Geometry: final body of the model. Coordinates: model frame, mm. A direction names the side the tool comes from. Round coordinates to 2 decimals unless told otherwise and drop trailing zeros. Order: outer loops, then holes, each group sorted by start corner. A loop starts at its lowest first (then second) coordinate and runs counter-clockwise, first axis right, second up. Notation, with made-up numbers: (15, -38.75) - (39, -38.75) arc R25 cw to (39, -12.75) - close; hole circle Ø8 at (-1, 14.25). An arc over 180 degrees is marked (long way). Put each result on its own line as item: value. Start each with the question number.
(1) Section C-C (z = 64). Output: boundary loops of the cut face in (x, y).
(2) Section D-D (x = 7). Output: boundary loops of the cut face in (y, z), and give its area (3 significant figures).
(3) Pull-direction query (X, two-part tool) for faces 1 (the face through (22.377, -63, 69)), 2 (the face through (67, -63, 22.86)), 3 (the face through (77.435, -63, 11)); classes: released by +X, released by -X, zero draft, split by the parting line, or undercut.
(4) Section B-B (x = 61). Output: boundary loops of the cut face in (y, z), and give its area (3 significant figures).
(5) Pin query (flat end, axial travel): P1, Ø7.5, axis at y = -72.5, z = 65.5, coming from the +X side; P2, Ø23, axis at x = 25, z = 38.5, coming from the -Y side; P3, Ø12.5, axis at y = -14.5, z = 49.5, coming from the +X side; P4, Ø1, axis at y = -26.5, z = 29.5, coming from the -X side. Return the tip coordinate at first contact, or that it passes through.
(6) Material intervals for L1, parallel to Z at x = 73.5, y = -66; L2, parallel to X at y = -58, z = 8.5; L3, parallel to Z at x = 9, y = -45, sorted ascending. Write a range as [from, to].
(7) Section A-A (y = -40.5). Output: boundary loops of the cut face in (x, z), and give its area (3 significant figures).
(8) Access query for faces 4 (the face through (24.278, -63, 10)), 5 (the face through (58.223, -63, 68)), 6 (the face through (13, -63, 20.32)), 7 (the face through (68, -63, 76.113)), 8 (the face through (68, -63, 60.945)). Directions: +Z, -Z, +X, -X, +Y, -Y. A direction counts if a zero-diameter tool reaches every point of the face in a straight line with its end or side. Return the directions, or none.
from build123d import *

# Parameters (mm, degrees)
F0_W     = 75.953597
F0_H     = 76.343752
F1_DEPTH = 25.4
F2_W     = 22.86
F2_H     = 20.32
F2_W_2   = 20.958833
F2_H_2   = 15.39883
F3_DEPTH = 76.2
F5_W     = 20.32
F5_H     = 22.86
F5_W_2   = 19.010187
F5_H_2   = 15.167706
F6_DEPTH = 76.2


with BuildPart() as f1:
    # F0 (on Front) → F1 (new body)
    with BuildSketch(Plane.XZ):
        with Locations((39.394597, 38.171876)):
            Rectangle(F0_W, F0_H)
    extrude(amount=F1_DEPTH)

    # F2 (on face) → F3 (join)
    with BuildSketch(Plane.XZ.offset(25.4)):
        with Locations((12.847799, 10.16)):
            Rectangle(F2_W, F2_H)
        with Locations((11.897215, 68.644337)):
            Rectangle(F2_W_2, F2_H_2)
    extrude(amount=F3_DEPTH)

    # F5 (on face) → F6 (join)
    with BuildSketch(Plane.XZ.offset(25.4)):
        with Locations((67.275393, 11.43)):
            Rectangle(F5_W, F5_H)
        with Locations((67.728057, 68.528775)):
            Rectangle(F5_W_2, F5_H_2)
    extrude(amount=F6_DEPTH)


solid = f1.part
Checks:
1. outline: (1.42, -101.6) - (22.38, -101.6) - (22.38, -25.4) - (58.22, -25.4) - (58.22, -101.6) - (77.23, -101.6) - (77.23, -25.4) - (77.37, -25.4) - (77.37, 0) - (1.42, 0) - close
2. outline: (-101.6, 0) - (0, 0) - (0, 76.34) - (-101.6, 76.34) - (-101.6, 60.94) - (-25.4, 60.94) - (-25.4, 20.32) - (-101.6, 20.32) - close
2. area: 4,660 mm²
3. face 1: undercut
3. face 2: zero draft
3. face 3: released by +X
4. outline: (-101.6, 0) - (0, 0) - (0, 76.34) - (-25.4, 76.34) - (-25.4, 76.11) - (-101.6, 76.11) - (-101.6, 60.94) - (-25.4, 60.94) - (-25.4, 22.86) - (-101.6, 22.86) - close
4. area: 4,840 mm²
5. P1: stops at x = 77.23
5. P2: stops at y = -25.4
5. P3: stops at x = 77.37
5. P4: passes through
6. L1: z = [0, 22.86], [60.94, 76.11]
6. L2: x = [1.42, 24.28], [57.12, 77.44]
6. L3: z = [0, 20.32], [60.94, 76.34]
7. outline: (1.42, 0) - (24.28, 0) - (24.28, 20.32) - (1.42, 20.32) - close; (1.42, 60.94) - (22.38, 60.94) - (22.38, 76.34) - (1.42, 76.34) - close; (57.12, 0) - (77.44, 0) - (77.44, 22.86) - (57.12, 22.86) - close; (58.22, 60.94) - (77.23, 60.94) - (77.23, 76.11) - (58.22, 76.11) - close
7. area: 1,540 mm²
8. face 4: +Z, -Z, -Y
8. face 5: +Z, -Y
8. face 6: -X, -Y
8. face 7: +Z, +X, -Y
8. face 8: +X, -X, -Y
